Here's how the part is built. I have some questions about the finished solid (model axes, mm). A direction names the side the tool comes from. Coordinates: 2 decimals unless noted, no trailing zeros. Order: outer loops, then holes, each group sorted by start corner. A loop starts at its lowest first (then second) coordinate and runs counter-clockwise, first axis right, second up. Notation, with made-up numbers: (76, -7) - (132, -7) arc R31 ccw to (132, 19) - close; hole circle Ø1 at (52, 56.5). An arc over 180 degrees is marked (long way). Answer as CSV lines item,"result". Start each with the question number.
Item 1: On a 3-axis mill with a long thin cutter (end or side, diameter ignored), from which of +Z, -Z, +X, -X, +Y, -Y can I reach the whole of each face in a straight line? I mean faces 1 (the face through (7, 0, 12)), 2 (the face through (7, 30, 13)), 3 (the face through (21, 20, 10)), 4 (the face through (17.47, 3.51, -1.48)). Say none if no direction works.
Item 2: Imagine slicing it at A-A on y = 15. List the corners of the cut face in (x, z) for me, and give its area (3 significant figures).
Item 3: I need wall thicknesses on line 1 (X direction, y = 7, z = 26); line 2 (Y direction, x = 30, z = 2.75); line 3 (Z direction, x = 8, y = 15). Which ranges of each line are inside material? Lowest first, please.
Item 4: I'm going to push flat-ended pins straight in: pin 1 (2 mm diameter, centred on x = 47.5, y = 27.5, fed in from +Z); pin 2 (14 mm diameter, centred on x = 51, z = 21, fed in from -Y); pin 3 (9 mm diameter, centred on x = 13, z = 14.5, fed in from +Y). Where does each tip first touch, or does it pass through?
Item 5: Imagine slicing it at B-B on z = 5.5. List the corners of the cut face in (x, y) for me (3 decimals), and give its area (3 significant figures).
Item 6: Imagine slicing it at D-D on x = 36. List the corners of the cut face in (y, z) for me.
Item 7: We'd pull the mould along X, two halves only. Please class faces 5 (the face through (30, -5, 5)), 6 (the face through (53, 30, 12)), 7 (the face through (50, 15, 25)), 8 (the face through (39.54, 12, 3.59)): pulls with the +X half, pulls with the -X half, needs draft (parallel to the pull), parting line crosses it, or undercut.
Item 8: Imagine slicing it at C-C on z = 14.5. List the corners of the cut face in (x, y) for me, and give its area (3 significant figures).
from build123d import *

# Parameters (mm, degrees)
F1_DEPTH  = 10
F2_R      = 10
F3_DEPTH  = 10.001
F4_R      = 17
F4_R_2    = 10
F5_DEPTH  = 3
F7_R      = 5
F8_DEPTH  = 10
F9_R      = 5
F10_DEPTH = 10


with BuildPart() as f1:
    # F0 (on Top) → F1 (new body)
    with BuildSketch(Plane.XY):
        with BuildLine():
            Line((42.5, 0), (17.5, 0))
            ThreePointArc((17.5, 0), (30, -5), (42.5, 0))
        make_face()
        with BuildLine():
            Line((0, 30), (0, 0))
            Line((0, 0), (17.5, 0))
            Line((17.5, 0), (42.5, 0))
            Line((42.5, 0), (60, 0))
            Line((60, 0), (60, 30))
            Line((60, 30), (42.5, 30))
            ThreePointArc((42.5, 30), (30, 35), (17.5, 30))
            Line((17.5, 30), (0, 30))
        make_face()
    extrude(amount=F1_DEPTH)

    # F2 (on face) → F3 (cut, through all)
    with BuildSketch(Plane.XY.offset(10)):
        with Locations((30, 15)):
            Circle(F2_R)
    extrude(amount=-F3_DEPTH, mode=Mode.SUBTRACT)

    # F4 (on face) → F5 (join)
    with BuildSketch(Plane(origin=(0, 0, 0), x_dir=(1, 0, 0), z_dir=(0, 0, -1))):
        with Locations((30, -15)):
            Circle(F4_R)
        with Locations((30, -15)):
            Circle(F4_R_2, mode=Mode.SUBTRACT)
    extrude(amount=F5_DEPTH)

    # F7 (on face) → F8 (join)
    with BuildSketch(Plane.YZ.offset(60)):
        with BuildLine():
            Line((30, 10), (30, 32))
            ThreePointArc((30, 32), (15, 17), (0, 32))
            Line((0, 32), (0, 10))
            Line((0, 10), (30, 10))
        make_face()
        with BuildLine():
            ThreePointArc((0, 32), (15, 17), (30, 32))
            ThreePointArc((30, 32), (15, 47), (0, 32))
        make_face()
        with Locations((15, 32)):
            Circle(F7_R, mode=Mode.SUBTRACT)
    extrude(amount=-F8_DEPTH)

    # F9 (on face) → F10 (join)
    with BuildSketch(Plane(origin=(0, 0, 0), x_dir=(0, -1, 0), z_dir=(-1, 0, 0))):
        with BuildLine():
            Line((0, 10), (0, 32))
            ThreePointArc((0, 32), (-15, 17), (-30, 32))
            Line((-30, 32), (-30, 10))
            Line((-30, 10), (0, 10))
        make_face()
        with BuildLine():
            ThreePointArc((-30, 32), (-15, 17), (0, 32))
            ThreePointArc((0, 32), (-15, 47), (-30, 32))
        make_face()
        with Locations((-15, 32)):
            Circle(F9_R, mode=Mode.SUBTRACT)
    extrude(amount=-F10_DEPTH)


solid = f1.part
Responses:
1,face 1,"+Z, -Z, -X, -Y"
1,face 2,"+Z, -Z, -X, +Y"
1,face 3,"+Z, +Y, -Y"
1,face 4,"-Z"
2,outline,"(0, 0) - (13, 0) - (13, -3) - (20, -3) - (20, 10) - (10, 10) - (10, 27) - (0, 27) - close; (0, 37) - (10, 37) - (10, 47) - (0, 47) - close; (40, -3) - (47, -3) - (47, 0) - (60, 0) - (60, 27) - (50, 27) - (50, 10) - (40, 10) - close; (50, 37) - (60, 37) - (60, 47) - (50, 47) - close"
2,area,"982 mm^2"
3,line 1,"x = 0 to 10, 50 to 60"
3,line 2,"y = -5 to 5, 25 to 35"
3,line 3,"z = 0 to 27, 37 to 47"
4,pin 1,"stops at z = 10"
4,pin 2,"stops at y = 0"
4,pin 3,"stops at y = 30"
5,outline,"(0, 0) - (17.5, 0) arc R18.125 ccw to (42.5, 0) - (60, 0) - (60, 30) - (42.5, 30) arc R18.125 ccw to (17.5, 30) - (0, 30) - close; hole circle Ø20 at (30, 15)"
5,area,"1,660 mm^2"
6,outline,"(-3.98, 0) - (-0.91, 0) - (-0.91, -3) - (7, -3) - (7, 10) - (-3.98, 10) - close; (23, -3) - (30.91, -3) - (30.91, 0) - (33.98, 0) - (33.98, 10) - (23, 10) - close"
7,face 5,"parting line crosses it"
7,face 6,"needs draft"
7,face 7,"undercut"
7,face 8,"undercut"
8,outline,"(0, 0) - (10, 0) - (10, 30) - (0, 30) - close; (50, 0) - (60, 0) - (60, 30) - (50, 30) - close"
8,area,"600 mm^2"
